Verification items for the finished model (mm, model axes). A direction names the side the tool comes from. Coordinates: 2 decimals unless noted, no trailing zeros. Order: outer loops, then holes, each group sorted by start corner. A loop starts at its lowest first (then second) coordinate and runs counter-clockwise, first axis right, second up.
Q1. Cross-section at C-C, the plane z = 19.5. Record the boundary of the cut face in (x, y).
Q2. Cross-section at A-A, the plane x = 0. Record the boundary of the cut face in (y, z), and give its area (3 significant figures).
Q3. Draft check along X on faces 1 (the cylindrical face through (-11.1, 0.07, 1.48)), 2 (the flat face through (0, 0, 0)), 3 (the cylindrical face through (15.929, 5.016, 13.378)). Enter one of: pulls with the +X half, pulls with the -X half, needs draft (parallel to the pull), parting line crosses it, or undercut.
Q4. Set-up check for faces 4 (the cylindrical face through (-0.54, -2.44, 30.95)), 5 (the flat face through (9, 0, 3)), 6 (the flat face through (0, 0, 38.05)): record each of +Z, -Z, +X, -X, +Y, -Y from which the full face is reachable in a straight line by a thin tool's end or side.
Q5. Cross-section at D-D, the plane y = -4.5. Record the boundary of the cut face in (x, z), and give its area (3 significant figures).
Q6. Cross-section at B-B, the plane y = -9.5. Record the boundary of the cut face in (x, z).
Q7. Thickness scan on line 1 (Y direction, x = 0, z = 0.9); line 2 (Z direction, x = -2, y = -13.5); line 3 (Z direction, x = -4.5, y = 12). Record the ranges inside material, lowest first.
Q8. Depth check by flat-ended pin: P1, Ø1, axis at x = 0.5, y = -10, coming from the -Z side; P2, Ø10, axis at x = -10.5, z = 6, coming from the +Y side; P3, Ø4, axis at x = -9.5, y = 0, coming from the +Z side. Enter the tip coordinate at first touch or a pass-through.
from build123d import *

# Parameters (mm, degrees)
SKETCH_1_R        = 13
SKETCH_1_R_2      = 1.6
EXTRUDE_228_DEPTH = 3
EXTRUDE_START     = 3
SKETCH_2_R        = 16.7
EXTRUDE_287_DEPTH = 21.05
M5_14MM_START     = 24.05
SKETCH_3_R        = 2.5
M5_14MM_DEPTH     = 14


with BuildPart() as part:
    # 草图1 → Extrude 228 (new body)
    with BuildSketch(Plane.XY):
        Circle(SKETCH_1_R)
        with Locations((-9.5, 0)):
            Circle(SKETCH_1_R_2, mode=Mode.SUBTRACT)
        with Locations((0, -9.5)):
            Circle(SKETCH_1_R_2, mode=Mode.SUBTRACT)
        with Locations((9.5, 0)):
            Circle(SKETCH_1_R_2, mode=Mode.SUBTRACT)
        with Locations((0, 9.5)):
            Circle(SKETCH_1_R_2, mode=Mode.SUBTRACT)
    extrude(amount=EXTRUDE_228_DEPTH)

    # 草图2 → Extrude 287 (add)
    with BuildSketch(Plane.XY.offset(EXTRUDE_START)):
        Circle(SKETCH_2_R)
    extrude(amount=EXTRUDE_287_DEPTH)

    # 草图3 → M5桨轴_外伸14mm (add)
    with BuildSketch(Plane.XY.offset(M5_14MM_START)):
        Circle(SKETCH_3_R)
    extrude(amount=M5_14MM_DEPTH)


solid = part.part
Check values:
1. outline: circle Ø33.4 at (0, 0)
2. outline: (-16.7, 3) - (-13, 3) - (-13, 0) - (-11.1, 0) - (-11.1, 3) - (-7.9, 3) - (-7.9, 0) - (7.9, 0) - (7.9, 3) - (11.1, 3) - (11.1, 0) - (13, 0) - (13, 3) - (16.7, 3) - (16.7, 24.05) - (2.5, 24.05) - (2.5, 38.05) - (-2.5, 38.05) - (-2.5, 24.05) - (-16.7, 24.05) - close
2. area: 832 mm2
3. face 1: undercut
3. face 2: needs draft
3. face 3: parting line crosses it
4. face 4: +Z
4. face 5: -Z
4. face 6: +Z, +X, -X, +Y, -Y
5. outline: (-16.08, 3) - (-12.2, 3) - (-12.2, 0) - (12.2, 0) - (12.2, 3) - (16.08, 3) - (16.08, 24.05) - (-16.08, 24.05) - close
5. area: 750 mm2
6. outline: (-13.73, 3) - (-8.87, 3) - (-8.87, 0) - (-1.6, 0) - (-1.6, 3) - (1.6, 3) - (1.6, 0) - (8.87, 0) - (8.87, 3) - (13.73, 3) - (13.73, 24.05) - (-13.73, 24.05) - close
7. line 1: y = -13 to -11.1, -7.9 to 7.9, 11.1 to 13
7. line 2: z = 3 to 24.05
7. line 3: z = 0 to 24.05
8. P1: stops at z = 3
8. P2: stops at y = 15.77
8. P3: stops at z = 24.05
